```python
from build123d import *

# Parameters (mm, degrees)
F0_W     = 101.6
F0_H     = 63.5
F1_DEPTH = 38.1
F2_W     = 50.8
F2_H     = 25.4
F3_DEPTH = 38.101
F4_DEPTH = 19.05


with BuildPart() as f1:
    # F0 (on Front) → F1 (new body)
    with BuildSketch(Plane.XZ):
        Rectangle(F0_W, F0_H)
    extrude(amount=F1_DEPTH)

    # F2 (on face) → F3 (cut, through all)
    with BuildSketch(Plane.XZ.offset(38.1)):
        with Locations((25.4, 0)):
            Rectangle(F2_W, F2_H)
    extrude(amount=-F3_DEPTH, mode=Mode.SUBTRACT)

    # F2 (on face) → F4 (cut)
    with BuildSketch(Plane.XZ.offset(38.1)):
        with Locations((25.4, 0)):
            Rectangle(F2_W, F2_H)
        Polygon((50.8, 31.75), (-25.4, 31.75), (-25.4, -31.75), (50.8, -31.75), (50.8, -12.7), (0, -12.7), (0, 12.7), (50.8, 12.7), align=None)
    extrude(amount=-F4_DEPTH, mode=Mode.SUBTRACT)


solid = f1.part
```
Could you check a few things on this model? Use its own coordinates, in mm. A direction names the side the tool comes from. Give positions to 0.01 mm unless a question says otherwise; leave off trailing zeros. Order: outer loops, then holes, each group sorted by start corner. A loop starts at its lowest first (then second) coordinate and runs counter-clockwise, first axis right, second up.
Q1. Suppose I cut it at D-D, the plane z = -24. Write out the boundary of the cut face in (x, y), and give its area (3 significant figures).
Q2. Suppose I cut it at A-A, the plane x = 31.5. Write out the boundary of the cut face in (y, z).
Q3. Suppose I cut it at B-B, the plane z = -3.5. Write out the boundary of the cut face in (x, y).
Q4. Suppose I cut it at C-C, the plane x = -8. Write out the boundary of the cut face in (y, z).
Q5. For faces 1 (the flat face through (-5, -19.05, 0)), 2 (the flat face through (-38, -38.1, 0)), 3 (the flat face through (0, -10, 0)), which set-ups out of +Z, -Z, +X, -X, +Y, -Y let a thin tool reach every point of the face, with its end or its side?
Q6. I'm going to push flat-ended pins straight in: P1, Ø1, axis at y = -33.5, z = -0.5, coming from the +X side; P2, Ø9.5, axis at y = -8, z = -4, coming from the +X side; P3, Ø8, axis at x = -8, z = -19, coming from the -Y side. Where does each tip first touch, or does it pass through?
Q7. If I drill on line 1 along Z through (x, y) = (6, -14.5); line 2 along X through (y, z) = (-22.5, -18); line 3 along Y through (x, z) = (28.5, 25), over which ranges is the centre line in solid material (lowest first)?
Q8. We'd pull the mould along Z, two halves only. Please class faces 4 (the flat face through (50.8, -9, -22)), 5 (the flat face through (-12, -15, 31.75)), 6 (the flat face through (25, -10, 12.7)), 7 (the flat face through (-12, -15, -31.75)): +Z half, -Z half, draft (parallel to the pull), parting line (faces both ways), or undercut.
Solution:
1. outline: (-50.8, -38.1) - (-25.4, -38.1) - (-25.4, -19.05) - (50.8, -19.05) - (50.8, 0) - (-50.8, 0) - close
1. area: 2,420 mm2
2. outline: (-19.05, -31.75) - (0, -31.75) - (0, -12.7) - (-19.05, -12.7) - close; (-19.05, 12.7) - (0, 12.7) - (0, 31.75) - (-19.05, 31.75) - close
3. outline: (-50.8, -38.1) - (-25.4, -38.1) - (-25.4, -19.05) - (0, -19.05) - (0, 0) - (-50.8, 0) - close
4. outline: (-19.05, -31.75) - (0, -31.75) - (0, 31.75) - (-19.05, 31.75) - close
5. face 1: +Z, -Z, +X, -Y
5. face 2: +Z, -Z, +X, -X, -Y
5. face 3: +X, +Y, -Y
6. P1: stops at x = -25.4
6. P2: stops at x = 0
6. P3: stops at y = -19.05
7. line 1: z = -31.75 to -12.7, 12.7 to 31.75
7. line 2: x = -50.8 to -25.4
7. line 3: y = -19.05 to 0
8. face 4: draft
8. face 5: +Z half
8. face 6: undercut
8. face 7: -Z half
